Check sheet for the modelled part. Datum: model origin and axes. Units: mm. Face numbers are marked on the shaded views. A direction names the side the tool comes from. Round coordinates to 2 decimals unless told otherwise and drop trailing zeros. Loops run counter-clockwise (first coordinate to the right, second up) from the corner with the lowest first, then second, coordinate; pieces in that order, holes last. Notation, with made-up numbers: (47, 78) -> (82, 78) arc R33 cw to (82, 107) -> close; hole circle Ø9 at (63, 66). An arc over 180 degrees is marked (long way). Return JSON: item names as keys, results as strings.
from build123d import *

# Parameters (mm, degrees)
BOSS_EXTRUDE1_DEPTH    = 30
BOSS_EXTRUDE3_DEPTH    = 30
CUT_EXTRUDE1_DEPTH     = 15
SKETCH7_R              = 5
CUT_EXTRUDE2_DEPTH     = 35
SKETCH8_R              = 10
BOSS_EXTRUDE4_DEPTH    = 10
SKETCH10_R             = 5
CUT_EXTRUDE6_DEPTH     = 10
SKETCH12_R             = 2.5
CUT_EXTRUDE7_DEPTH     = 10
SKETCH13_R             = 5
CUT_EXTRUDE8_DEPTH     = 10
M12_TAPPED_HOLE1_D     = 10.2
M12_TAPPED_HOLE1_DEPTH = 15
M12_TAPPED_HOLE1_TIP   = 3.064389157


with BuildPart() as part:
    # Sketch1 → Boss-Extrude1 (new body)
    with BuildSketch(Plane.XY):
        with BuildLine():
            Line((-40, 30), (-40, 15))
            Line((-40, 15), (-30, 15))
            ThreePointArc((-30, 15), (-15, 0), (-30, -15))
            Line((-30, -15), (-40, -15))
            Line((-40, -15), (-40, -30))
            Line((-40, -30), (0, -30))
            ThreePointArc((0, -30), (30, 0), (0, 30))
            Line((0, 30), (-40, 30))
        make_face()
    extrude(amount=BOSS_EXTRUDE1_DEPTH)

    # Sketch5 → Boss-Extrude3 (add)
    with BuildSketch(Plane.XY.offset(30)):
        with BuildLine():
            Line((-30, 15), (-35, 15))
            Line((-35, 15), (-35, -15))
            Line((-35, -15), (-30, -15))
            ThreePointArc((-30, -15), (-15, 0), (-30, 15))
        make_face()
    extrude(amount=-BOSS_EXTRUDE3_DEPTH)

    # Sketch6 → Cut-Extrude1 (cut)
    with BuildSketch(Plane.XY.offset(30)):
        with BuildLine():
            Line((-35, 15), (-30, 15))
            ThreePointArc((-30, 15), (-14.999999991, 0.000506597), (-29.998986771, -15))
            Line((-29.998986771, -15), (-35, -15))
            Line((-35, -15), (-35, 15))
        make_face()
    extrude(amount=-CUT_EXTRUDE1_DEPTH, mode=Mode.SUBTRACT)

    # Sketch7 → Cut-Extrude2 (cut)
    with BuildSketch(Plane.XY.offset(15)):
        with Locations((-25, 0)):
            Circle(SKETCH7_R)
    extrude(amount=-CUT_EXTRUDE2_DEPTH, mode=Mode.SUBTRACT)

    # Sketch8 → Boss-Extrude4 (add)
    with BuildSketch(Plane.XY.offset(30)):
        Circle(SKETCH8_R)
    extrude(amount=BOSS_EXTRUDE4_DEPTH)

    # Sketch10 → Cut-Extrude6 (cut)
    with BuildSketch(Plane.XY.offset(30)):
        with Locations((15, 15)):
            Circle(SKETCH10_R)
        with Locations((15, -15)):
            Circle(SKETCH10_R)
    extrude(amount=-CUT_EXTRUDE6_DEPTH, mode=Mode.SUBTRACT)

    # Sketch12 → Cut-Extrude7 (cut)
    with BuildSketch(Plane.XY.offset(20)):
        with Locations((15, 15)):
            Circle(SKETCH12_R)
        with Locations((15, -15)):
            Circle(SKETCH12_R)
    extrude(amount=-CUT_EXTRUDE7_DEPTH, mode=Mode.SUBTRACT)

    # Sketch13 → Cut-Extrude8 (cut)
    with BuildSketch(Plane(origin=(0, 0, 0), x_dir=(-1, 0, 0), z_dir=(0, 0, -1))):
        with Locations((-15, 15)):
            Circle(SKETCH13_R)
        with Locations((-15, -15)):
            Circle(SKETCH13_R)
    extrude(amount=-CUT_EXTRUDE8_DEPTH, mode=Mode.SUBTRACT)

    # M12 Tapped Hole1
    with Locations(Plane.XY.offset(40)):
        with Locations((0, 0)):
            Hole(M12_TAPPED_HOLE1_D / 2, depth=M12_TAPPED_HOLE1_DEPTH)
            with Locations((0, 0, -(M12_TAPPED_HOLE1_DEPTH + M12_TAPPED_HOLE1_TIP / 2))):  # 118° drill point
                Cone(0, M12_TAPPED_HOLE1_D / 2, M12_TAPPED_HOLE1_TIP, mode=Mode.SUBTRACT)


solid = part.part
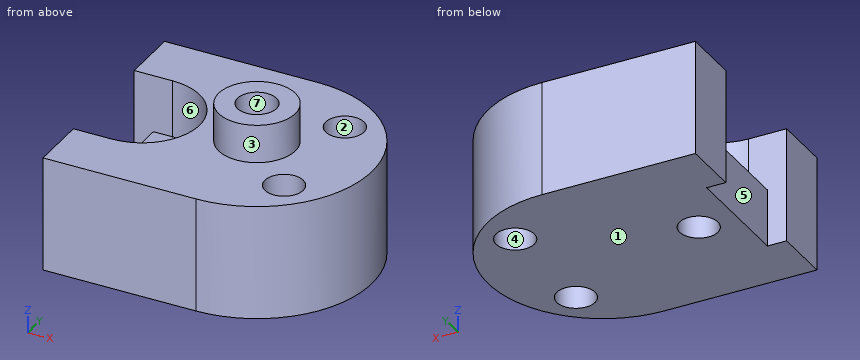
Q1. Material ranges on line 1 (Y direction, x = -25, z = 3); line 2 (Y direction, x = 15, z = 5); line 3 (Z direction, x = -20.5, y = -8.5), recorded low to high.
Results list:
{"line 1": "-30 to -5, 5 to 30", "line 2": "-25.98 to -20, -10 to 10, 20 to 25.98", "line 3": "0 to 15"}
Q2. Draft check along X on the marked faces 1, 2 and 3. Enter one of: released by +X, released by -X, zero draft, split by the parting line, or undercut.
Results list:
{"face 1": "zero draft", "face 2": "undercut", "face 3": "split by the parting line"}
Q3. Section check A-A (z = 28.5). Record the boundary of the cut face in (x, y).
Results list:
{"outline": "(-40, -30) -> (0, -30) arc R30 ccw to (0, 30) -> (-40, 30) -> (-40, 15) -> (-30, 15) arc R15 cw to (-30, -15) -> (-40, -15) -> close; hole circle Ø10.2 at (0, 0); hole circle Ø10 at (15, -15); hole circle Ø10 at (15, 15)"}
Q4. Go/stop test with flat-tipped pins: pin 1 (6.5 mm diameter, centred on x = 15, y = -15, fed in from -Z); pin 2 (3 mm diameter, centred on x = -28.5, y = 8.5, fed in from +Z); pin 3 (1 mm diameter, centred on y = -5, z = 7.5, fed in from +X). Record where each tip stops, or that it passes through.
Results list:
{"pin 1": "z = 10", "pin 2": "z = 15", "pin 3": "x = 29.66"}
Q5. Section check C-C (y = -7). Record the boundary of the cut face in (x, z).
Results list:
{"outline": "(-35, 0) -> (29.17, 0) -> (29.17, 30) -> (7.14, 30) -> (7.14, 40) -> (-7.14, 40) -> (-7.14, 30) -> (-16.73, 30) -> (-16.73, 15) -> (-35, 15) -> close"}
Q6. Section check D-D (x = -25). Record the boundary of the cut face in (y, z).
Results list:
{"outline": "(-30, 0) -> (-5, 0) -> (-5, 15) -> (-14.14, 15) -> (-14.14, 30) -> (-30, 30) -> close; (5, 0) -> (30, 0) -> (30, 30) -> (14.14, 30) -> (14.14, 15) -> (5, 15) -> close"}
Q7. Tool access check on the marked faces 4, 5, 6 and 7. Record the directions out of +Z, -Z, +X, -X, +Y, -Y that give a thin tool (end or side, any length) a straight path to the whole face; none if there is none.
Results list:
{"face 4": "-Z", "face 5": "+Z, -Z, -X", "face 6": "+Z, -X", "face 7": "+Z"}
Q8. Section check B-B (x = 15). Record the boundary of the cut face in (y, z).
Results list:
{"outline": "(-25.98, 0) -> (-20, 0) -> (-20, 10) -> (-17.5, 10) -> (-17.5, 20) -> (-20, 20) -> (-20, 30) -> (-25.98, 30) -> close; (-12.5, 10) -> (-10, 10) -> (-10, 0) -> (10, 0) -> (10, 10) -> (12.5, 10) -> (12.5, 20) -> (10, 20) -> (10, 30) -> (-10, 30) -> (-10, 20) -> (-12.5, 20) -> close; (17.5, 10) -> (20, 10) -> (20, 0) -> (25.98, 0) -> (25.98, 30) -> (20, 30) -> (20, 20) -> (17.5, 20) -> close"}
